Work out the finished part from the listing and answer in its coordinate system (mm). A direction names the side the tool comes from. Round coordinates to 2 decimals unless told otherwise and drop trailing zeros. Loops run counter-clockwise (first coordinate to the right, second up) from the corner with the lowest first, then second, coordinate; pieces in that order, holes last.
```python
from build123d import *

# Parameters (mm, degrees)
SKETCH1_R           = 60
BOSS_EXTRUDE1_DEPTH = 15
SKETCH2_R           = 4.175
CUT_EXTRUDE1_DEPTH  = 10
SKETCH3_R           = 2.75
CUT_EXTRUDE2_DEPTH  = 87.168439698
SKETCH4_R           = 17.4625
CUT_EXTRUDE3_DEPTH  = 87.168439698
SKETCH5_R           = 6.5
CUT_EXTRUDE4_DEPTH  = 10


with BuildPart() as part:
    # Sketch1 → Boss-Extrude1 (new body)
    with BuildSketch(Plane(origin=(0, 0, 0), x_dir=(1, 0, 0), z_dir=(0, 1, 0))):
        with Locations(Location((0, 0, 0), (0, 0, 270))):
            Circle(SKETCH1_R)
    extrude(amount=BOSS_EXTRUDE1_DEPTH)

    # Sketch2 → Cut-Extrude1 (cut)
    with BuildSketch(Plane(origin=(0, 15, 0), x_dir=(1, 0, 0), z_dir=(0, 1, 0))):
        with Locations(Location((45, 0, 0), (0, 0, 270))):
            Circle(SKETCH2_R)
        with Locations(Location((0, -45, 0), (0, 0, 270))):
            Circle(SKETCH2_R)
        with Locations(Location((-45, 0, 0), (0, 0, 270))):
            Circle(SKETCH2_R)
        with Locations(Location((0, 45, 0), (0, 0, 270))):
            Circle(SKETCH2_R)
    extrude(amount=-CUT_EXTRUDE1_DEPTH, mode=Mode.SUBTRACT)

    # Sketch3 → Cut-Extrude2 (cut, through all)
    with BuildSketch(Plane.XZ):
        with Locations(Location((34.280536752, -34.280536752, 0), (0, 0, 270))):
            Circle(SKETCH3_R)
        with Locations(Location((-34.280536752, -34.280536752, 0), (0, 0, 270))):
            Circle(SKETCH3_R)
        with Locations(Location((-34.280536752, 34.280536752, 0), (0, 0, 270))):
            Circle(SKETCH3_R)
        with Locations(Location((34.280536752, 34.280536752, 0), (0, 0, 270))):
            Circle(SKETCH3_R)
    extrude(amount=-CUT_EXTRUDE2_DEPTH, mode=Mode.SUBTRACT)

    # Sketch4 → Cut-Extrude3 (cut, through all)
    with BuildSketch(Plane.XZ):
        with Locations(Location((0, 0, 0), (0, 0, 270))):
            Circle(SKETCH4_R)
    extrude(amount=-CUT_EXTRUDE3_DEPTH, mode=Mode.SUBTRACT)

    # Sketch5 → Cut-Extrude4 (cut)
    with BuildSketch(Plane(origin=(0, 15, 0), x_dir=(1, 0, 0), z_dir=(0, 1, 0))):
        with Locations(Location((-34.280536752, 34.280536752, 0), (0, 0, 270))):
            Circle(SKETCH5_R)
        with Locations(Location((34.280536752, 34.280536752, 0), (0, 0, 270))):
            Circle(SKETCH5_R)
        with Locations(Location((34.280536752, -34.280536752, 0), (0, 0, 270))):
            Circle(SKETCH5_R)
        with Locations(Location((-34.280536752, -34.280536752, 0), (0, 0, 270))):
            Circle(SKETCH5_R)
    extrude(amount=-CUT_EXTRUDE4_DEPTH, mode=Mode.SUBTRACT)


solid = part.part
```
1. Which of the six approach directions +Z, -Z, +X, -X, +Y, -Y give full straight-line access (tool end or side, diameter ignored) to faces 1 (the face through (36.139, 2.465, -32.254)), 2 (the face through (34.566, 10.07, 27.787))?
Answer key:
face 1: +Y, -Y
face 2: +Y
2. Find section C-C (x = -47). Write down the section's boundary in (y, z).
Answer key:
outline: (0, -37.3) - (15, -37.3) - (15, -3.66) - (5, -3.66) - (5, 3.66) - (15, 3.66) - (15, 37.3) - (0, 37.3) - close
3. Find section D-D (y = 11.5). Give the number of separate pieces and of enclosed holes in the cut face, then the cut area to 3 significant figures.
Answer key:
separate pieces: 1
enclosed holes: 9
area: 9,600 mm2
4. Determine the mould class of faces 3 (the face through (2.64, 7.4, -59.94)), 4 (the face through (-1.599, 10.07, 48.857)), 5 (the face through (-12.5, 15, 12.5)) for opening direction Z: +Z half, -Z half, draft (parallel to the pull), parting line (faces both ways), or undercut.
Answer key:
face 3: parting line
face 4: undercut
face 5: draft
5. Consider probe 1 along X at (y, z) = (10.5, 0) (1 decimal); probe 2 along Z at (x, y) = (32, 14); probe 3 along Z at (x, y) = (32.5, 5.5). Determine where each line is inside the solid, lowest interval first.
Answer key:
probe 1: x = -60 to -49.2, -40.8 to -17.5, 17.5 to 40.8, 49.2 to 60
probe 2: z = -50.75 to -40.37, -28.19 to 28.19, 40.37 to 50.75
probe 3: z = -50.44 to -40.53, -28.03 to 28.03, 40.53 to 50.44
6. Find section B-B (z = 0). Write down the section's boundary in (x, y) (1 decimal).
Answer key:
outline: (-60, 0) - (-17.5, 0) - (-17.5, 15) - (-40.8, 15) - (-40.8, 5) - (-49.2, 5) - (-49.2, 15) - (-60, 15) - close; (17.5, 0) - (60, 0) - (60, 15) - (49.2, 15) - (49.2, 5) - (40.8, 5) - (40.8, 15) - (17.5, 15) - close
7. Find section A-A (x = 0). Write down the section's boundary in (y, z) (1 decimal).
Answer key:
outline: (0, -60) - (15, -60) - (15, -49.2) - (5, -49.2) - (5, -40.8) - (15, -40.8) - (15, -17.5) - (0, -17.5) - close; (0, 17.5) - (15, 17.5) - (15, 40.8) - (5, 40.8) - (5, 49.2) - (15, 49.2) - (15, 60) - (0, 60) - close
8. Given pin 1 (4 mm diameter, centred on y = 11.5, z = 5.5, fed in from -X); pin 2 (5 mm diameter, centred on x = 30, y = 4, fed in from -Z); pin 3 (4 mm diameter, centred on x = -46, z = 0, fed in from +Y); pin 4 (3.5 mm diameter, centred on x = 34.28, z = -34.28, fed in from -Y), each flat-ended and moving along its own axis, determine where each tip first touches the part or whether it passes through.
Answer key:
pin 1: stops at x = -59.9
pin 2: stops at z = -53.33
pin 3: stops at y = 5
pin 4: passes through
